```python
from build123d import *

# Parameters (mm, degrees)
F0_W     = 300
F0_H     = 300
F1_DEPTH = 150
F2_R     = 100
F3_DEPTH = 10
F4_R     = 99
F5_DEPTH = 10


with BuildPart() as f1:
    # F0 (on Top) → F1 (new body, symmetric)
    with BuildSketch(Plane.XY):
        Rectangle(F0_W, F0_H)
    extrude(amount=F1_DEPTH, both=True)

    # F2 (on face) → F3 (cut)
    with BuildSketch(Plane.XY.offset(150)):
        Circle(F2_R)
    extrude(amount=-F3_DEPTH, mode=Mode.SUBTRACT)

    # F4 (on face) → F5 (join)
    with BuildSketch(Plane.XY.offset(140)):
        Circle(F4_R)
    extrude(amount=F5_DEPTH)


solid = f1.part
```
Here's how the part is built. I have some questions about the finished solid (model axes, mm). A direction names the side the tool comes from. Round coordinates to 2 decimals unless told otherwise and drop trailing zeros. Answer as CSV lines item,"result".
1. If I drill on L1, parallel to Y at x = 0, z = 147, over which ranges is the centre line in solid material (lowest first)?
Final values:
L1,"y = -150 to -100, -99 to 99, 100 to 150"
2. Thinking about a two-plate mould opening in Y: for faces 3 (the face through (-1, 1, 150)), 4 (the face through (-97, 23, 140)), 5 (the face through (-2, 150, 2)), which applies, released by +Y, released by -Y, zero draft, split by the parting line, or undercut?
Final values:
face 3,"zero draft"
face 4,"undercut"
face 5,"released by +Y"
3. Which directions (+Z, -Z, +X, -X, +Y, -Y) give clear straight access to the entire face, cutting with the end or side of a thin tool? Please do faces 1 (the face through (-12.888, 98.158, 144.93)), 2 (the face through (-2, 2, -150)).
Final values:
face 1,"+Z"
face 2,"-Z, +X, -X, +Y, -Y"
